The listing builds one solid part. Answer for the finished solid, in the listing's coordinates (mm). A direction names the side the tool comes from. Round coordinates to 2 decimals unless told otherwise and drop trailing zeros. Order: outer loops, then holes, each group sorted by start corner. A loop starts at its lowest first (then second) coordinate and runs counter-clockwise, first axis right, second up. Notation, with made-up numbers: M -38.75,-31 L -23.75,-31 A13 ccw -23.75,-26 Z; hole C -11,53.5 d4. An arc over 180 degrees is marked long. Put each result on its own line as item: value. Start each with the question number.
1. The mould has two halves that part along Z. Classify faces 6 (the face through (2, 22, 0)), 7 (the face through (2.535, -1.917, 37.079)), 8 (the face through (2.46, 47.19, 20.78)): +Z half, -Z half, draft (parallel to the pull), parting line (faces both ways), or undercut.
2. The part is cut by section B-B (z = 47.5). Give the vertices of the cut face in (x, y).
3. Each of these flat-tipped pins is pushed along its axis until it touches: pin 1 Ø0.9 at (x, y) = (1.5, 6) entering from +Z; pin 2 Ø1.5 at (x, y) = (3.5, 9.5) entering from +Z; pin 3 Ø2.5 at (x, z) = (3, 3.5) entering from -Y. Where does it stop, or does it pass through?
4. The part is cut by section A-A (y = 6). Give the vertices of the cut face in (x, z).
5. The part is cut by section C-C (y = 30). Give the vertices of the cut face in (x, z), then the cut area to 3 significant figures.
6. Consider line 1 (Z direction, x = 3.3, y = 4); line 2 (Y direction, x = 2.55, z = 4.5); line 3 (Y direction, x = 0.2, z = 8). Determine where each line is inside the solid, lowest interval first.
7. Which of the six approach directions +Z, -Z, +X, -X, +Y, -Y give full straight-line access (tool end or side, diameter ignored) to faces 1 (the face through (2.535, -21.168, 33.954)), 2 (the face through (2, 0, 11)), 3 (the face through (5, 0.4, 19.4)), 4 (the face through (3, 10, 5.5)), 5 (the face through (2.46, -8.8, 41.16))?
from build123d import *

# Parameters (mm, degrees)
BOSS_EXTRUDE1_DEPTH = 5
CUT_EXTRUDE1_DEPTH  = 73.173788448
CHAMFER1_SIZE       = 3
FILLET1_R           = 5


with BuildPart() as part:
    # Sketch1 → Boss-Extrude1 (new body)
    with BuildSketch(Plane(origin=(0, 0, 0), x_dir=(0, 0, -1), z_dir=(1, 0, 0))):
        Polygon((0, 0), (-14, 0), (-14, 2), (-19, 2), (-19, -50), (-51.807873329, -38.058910659), (-20, 49.332503075), (0, 49.332503075), align=None)
    extrude(amount=BOSS_EXTRUDE1_DEPTH)

    # Sketch2 → Cut-Extrude1 (cut, through all)
    with BuildSketch(Plane(origin=(5, 0, 0), x_dir=(0, 0, -1), z_dir=(1, 0, 0))):
        Polygon((-21.539090645, 45.103886281), (-16.840627541, 43.393785564), (-16.413102362, 44.56840134), (-13.5940245, 43.54234091), (-14.021549679, 42.367725134), (-11.202471816, 41.341664704), (-12.228532246, 38.522586842), (-15.047610109, 39.548647272), (-15.475135288, 38.374031496), (-18.29421315, 39.400091926), (-17.866687971, 40.574707702), (-22.565151075, 42.284808419), align=None)
        Polygon((-43.770399961, -15.97613407), (-44.796460391, -18.795211932), (-40.097997287, -20.505312649), (-40.525522466, -21.679928425), (-37.706444604, -22.705988855), (-37.278919425, -21.531373079), (-34.459841562, -22.557433509), (-33.433781132, -19.738355647), (-36.252858995, -18.712295217), (-35.825333816, -17.537679441), (-38.644411678, -16.511619011), (-39.071936857, -17.686234787), align=None)
        Polygon((-27.866463296, 27.719572796), (-38.46908774, -1.410898448), (-35.650009877, -2.436958878), (-25.047385434, 26.693512366), align=None)
        Polygon((-8.5, 0), (-8.5, 5), (-9.75, 5), (-9.75, 8), (-8.5, 8), (-8.5, 11), (-5.5, 11), (-5.5, 8), (-4.25, 8), (-4.25, 5), (-5.5, 5), (-5.5, 0), align=None)
    extrude(amount=-CUT_EXTRUDE1_DEPTH, mode=Mode.SUBTRACT)

    # Chamfer1
    chamfer1_edges = [part.edges().sort_by_distance(p)[0] for p in [
        (2.5, -38.058910659, 51.807873329),
    ]]
    chamfer(chamfer1_edges, length=CHAMFER1_SIZE)

    # Fillet1
    fillet1_edges = [part.edges().sort_by_distance(p)[0] for p in [
        (2.5, 49.332503075, 0),
    ]]
    fillet(fillet1_edges, radius=FILLET1_R)


solid = part.part
Resolved:
1. face 6: -Z half
1. face 7: undercut
1. face 8: +Z half
2. outline: M 0,-39.63 L 5,-39.63 L 5,-26.22 L 0,-26.22 Z
3. pin 1: z = 32.74
3. pin 2: z = 31.58
3. pin 3: y = 0
4. outline: M 0,0 L 5,0 L 5,4.25 L 0,4.25 Z; M 0,9.75 L 5,9.75 L 5,32.58 L 0,32.58 Z
5. outline: M 0,0 L 5,0 L 5,27.04 L 0,27.04 Z
5. area: 135 mm2
6. line 1: 0 to 5.5, 8.5 to 33.31
6. line 2: 0 to 5, 8 to 49.31
6. line 3: 11 to 49.33
7. face 1: +X, -X
7. face 2: -Z, +X, -X, -Y
7. face 3: +Z, -Z, +X, +Y, -Y
7. face 4: +X, -X, -Y
7. face 5: +Z, +X, -X, +Y
